The listing builds one solid part. Answer for the finished solid, in the listing's coordinates (mm). Round coordinates to 2 decimals unless told otherwise and drop trailing zeros. Order: outer loops, then holes, each group sorted by start corner. A loop starts at its lowest first (then second) coordinate and runs counter-clockwise, first axis right, second up. Notation, with made-up numbers: (32.25, -14) -> (75.25, -14) arc R20 ccw to (75.25, 19) -> close; hole circle Ø7 at (-9, 10.25). An arc over 180 degrees is marked (long way). Answer in a Markdown table with one row per item. Add a question column.
Autodesk Inventor part; units mm, degrees
ref_plane "YZ Plane" through (0, 0, 0) normal (1, 0, 0) x (0, 1, 0)
ref_plane "XZ Plane" through (0, 0, 0) normal (0, 1, 0) x (-1, 0, 0)
ref_plane "XY Plane" through (0, 0, 0) normal (0, 0, 1) x (1, 0, 0)
sketch "Sketch1" plane through (0, 0, 0) normal (0, 0, 1) x (1, 0, 0)
  line L0 (93.85, -64.2699) -> (-93.85, -64.2699)
  line L1 (-93.85, -64.2699) -> (-93.85, 55.2301)
  line L2 (-93.85, 55.2301) -> (93.85, 55.2301)
  line L3 (93.85, 55.2301) -> (93.85, -64.2699)
  line L4 (93.85, -64.2699) -> (-93.85, 55.2301) construction
  line L5 (-93.85, -64.2699) -> (93.85, 55.2301) construction
  point P0 (0, 0)
  point P1 (0, -4.5199)
  dimension "d0" = 187.7
  dimension "d1" = 119.5
extrude "Extrusion1" add sketch "Sketch1" along normal mid plane 2.5
hole "Hole2" at (-88.85, -59.3199, 1.25) direction (0, 0, -1) diameter 4 end through all countersink diameter 7 countersink angle 90
hole "Hole3" at (0, -59.2699, 1.25) direction (0, 0, -1) diameter 4 end through all countersink diameter 7 countersink angle 90
hole "Hole4" at (88.9, -59.2699, 1.25) direction (0, 0, -1) diameter 4 end through all countersink diameter 7 countersink angle 90
hole "Hole5" at (-88.9, 50.2301, 1.25) direction (0, 0, -1) diameter 4 end through all countersink diameter 7 countersink angle 90
hole "Hole6" at (0, 50.2301, 1.25) direction (0, 0, -1) diameter 4 end through all countersink diameter 7 countersink angle 90
hole "Hole7" at (88.9, 50.2301, 1.25) direction (0, 0, -1) diameter 4 end through all countersink diameter 7 countersink angle 90
hole "Hole8" at (76.35, -38.2699, 1.25) direction (0, 0, -1) diameter 4 end through all
hole "Hole9" at (76.35, 30.7301, 1.25) direction (0, 0, -1) diameter 4 end through all
hole "Hole10" at (-75.65, -38.2699, 1.25) direction (0, 0, -1) diameter 4 end through all
hole "Hole11" at (-75.65, 30.7301, 1.25) direction (0, 0, -1) diameter 4 end through all
sketch "Sketch5" plane through (0, 0, 1.25) normal (0, 0, 1) x (1, 0, 0)
  circle A0 centre (76.35, -38.2699) radius 2
  line L0 (93.85, -64.2699) -> (93.85, 55.2301)
  line L1 (-0.65, -21.7699) -> (85.35, -21.7699)
  line L2 (85.35, -21.7699) -> (85.35, -32.7699)
  line L3 (85.35, -32.7699) -> (-0.65, -32.7699)
  line L4 (-0.65, -32.7699) -> (-0.65, -21.7699)
  point P0 (0, 0)
  dimension "d120" = 8.5
  dimension "d121" = 5.5
  dimension "d122" = 11
  dimension "d123" = 86
extrude "Cut1" cut sketch "Sketch5" along normal through all both and the other way through all contours L1 L2 L3 L4
pattern_linear "Rectangular Pattern1" count 2 spacing 45.5 along (0, 1, 0) of "Cut1"
sketch "Sketch6" plane through (0, 0, 1.25) normal (0, 0, 1) x (1, 0, 0)
  line L0 (85.35, 23.7301) -> (85.35, 12.7301)
  line L1 (85.35, 12.7301) -> (-0.65, 12.7301)
  line L2 (5.85, 43.4801) -> (78.85, 43.4801)
  line L3 (78.85, 43.4801) -> (78.85, 33.2301)
  line L4 (78.85, 33.2301) -> (5.85, 33.2301)
  line L5 (5.85, 33.2301) -> (5.85, 43.4801)
  line L6 (-0.65, 23.7301) -> (-0.65, 12.7301)
  line L7 (-0.65, 12.7301) -> (85.35, 12.7301)
  line L8 (85.35, 12.7301) -> (85.35, 23.7301)
  line L9 (85.35, 23.7301) -> (-0.65, 23.7301)
  line L10 (-0.65, -21.7699) -> (-0.65, -32.7699)
  line L11 (-0.65, -32.7699) -> (85.35, -32.7699)
  line L12 (85.35, -32.7699) -> (85.35, -21.7699)
  line L13 (85.35, -21.7699) -> (-0.65, -21.7699)
  circle A0 centre (-75.65, 30.7301) radius 2
  circle A1 centre (-75.65, -38.2699) radius 2
  circle A2 centre (76.35, 30.7301) radius 2
  circle A3 centre (76.35, -38.2699) radius 2
  line L14 (-93.85, -64.2699) -> (-93.85, 55.2301)
  line L15 (-93.85, 55.2301) -> (93.85, 55.2301)
  line L16 (93.85, 55.2301) -> (93.85, -64.2699)
  line L17 (93.85, -64.2699) -> (-93.85, -64.2699)
  circle A4 centre (-88.85, -59.3199) radius 3.5
  circle A5 centre (0, -59.2699) radius 3.5
  circle A6 centre (88.9, -59.2699) radius 3.5
  circle A7 centre (-88.9, 50.2301) radius 3.5
  circle A8 centre (0, 50.2301) radius 3.5
  circle A9 centre (88.9, 50.2301) radius 3.5
  point P0 (0, 0)
  dimension "d129" = 6.5
  dimension "d130" = 20.5
  dimension "d131" = 73
  dimension "d132" = 10.25
extrude "Cut2" cut sketch "Sketch6" against normal through all contours L2 L3 L4 L5
hole "Hole12" at (5.85, 43.4801, 1.25) direction (0, 0, -1) diameter 3 end through all
hole "Hole13" at (78.85, 43.4801, 1.25) direction (0, 0, -1) diameter 3 end through all
hole "Hole14" at (5.85, 33.2301, 1.25) direction (0, 0, -1) diameter 3 end through all
hole "Hole16" at (78.85, 33.2301, 1.25) direction (0, 0, -1) diameter 3 end through all
hole "Hole17" at (-0.65, 23.7301, 1.25) direction (0, 0, -1) diameter 3 end through all
hole "Hole18" at (-0.65, 12.7301, 1.25) direction (0, 0, -1) diameter 3 end through all
hole "Hole19" at (85.35, 12.7301, 1.25) direction (0, 0, -1) diameter 3 end through all
hole "Hole20" at (85.35, 23.7301, 1.25) direction (0, 0, -1) diameter 3 end through all
hole "Hole21" at (-0.65, -21.7699, 1.25) direction (0, 0, -1) diameter 3 end through all
hole "Hole22" at (-0.65, -32.7699, 1.25) direction (0, 0, -1) diameter 3 end through all
hole "Hole23" at (85.35, -21.7699, 1.25) direction (0, 0, -1) diameter 3 end through all
hole "Hole24" at (85.35, -32.7699, 1.25) direction (0, 0, -1) diameter 3 end through all
equation "\"d124\" = Thickness"
equation "\"d133\" = Thickness"
equation "\"d142\" = Thickness"
equation "\"d151\" = Thickness"
equation "\"d160\" = Thickness"
equation "\"d178\" = Thickness"
equation "\"d187\" = Thickness"
equation "\"d196\" = Thickness"
equation "\"d205\" = Thickness"
equation "\"d214\" = Thickness"
equation "\"d223\" = Thickness"
equation "\"d232\" = Thickness"
equation "\"d241\" = Thickness"
equation "\"d250\" = Thickness"
equation "\"BendRadius\" = Thickness"
equation "\"BendReliefWidth\" = Thickness"
equation "\"BendReliefDepth\" = 0.5 * Thickness"
equation "\"CornerReliefSize\" = 4 * Thickness"
equation "\"MinimumRemnant\" = 2 * Thickness"
equation "\"TransitionRadius\" = BendRadius"
equation "\"JacobiRadiusSize\" = Thickness"
equation "\"GapSize\" = Thickness"
properties part number "Driver4BusV11Top"
1. The mould has two halves that part along Y. Classify faces 1 (the flat face through (-1, -4, 1.25)), 2 (the cylindrical face through (78.124, 29.807, -0.018)): released by +Y, released by -Y, zero draft, split by the parting line, or undercut.
2. The part is cut by section B-B (y = 18). Give the vertices of the cut face in (x, z), then the cut area to 3 significant figures.
3. The part is cut by section C-C (x = -75.65). Give the vertices of the cut face in (y, z), then the cut area to 3 significant figures.
4. Each of these flat-tipped pins is pushed along its axis until it touches: pin 1 (3.5 mm diameter, centred on x = -88.85, y = -59.32, fed in from -Z); pin 2 (4 mm diameter, centred on x = -0.65, y = -32.77, fed in from +Z); pin 3 (4.5 mm diameter, centred on x = 0, y = 50.23, fed in from +Z). Where does it stop, or does it pass through?
5. Straight lines are drawn through the part: line 1 along Y through (x, z) = (65.5, 1.1); line 2 along Y through (x, z) = (-75.65, -0.3); line 3 along Y through (x, z) = (0, -1). For each, find the intervals that lie inside material, in ascending order.
6. The part is cut by section D-D (x = 88.9). Give the vertices of the cut face in (y, z).
7. The part is cut by section A-A (x = 45). Give the vertices of the cut face in (y, z).
Report:
| question | item | result |
|---|---|---|
| 1 | face 1 | zero draft |
| 1 | face 2 | undercut |
| 2 | outline | (-93.85, -1.25) -> (-0.65, -1.25) -> (-0.65, 1.25) -> (-93.85, 1.25) -> close; (85.35, -1.25) -> (93.85, -1.25) -> (93.85, 1.25) -> (85.35, 1.25) -> close |
| 2 | area | 254 mm^2 |
| 3 | outline | (-64.27, -1.25) -> (-40.27, -1.25) -> (-40.27, 1.25) -> (-64.27, 1.25) -> close; (-36.27, -1.25) -> (28.73, -1.25) -> (28.73, 1.25) -> (-36.27, 1.25) -> close; (32.73, -1.25) -> (55.23, -1.25) -> (55.23, 1.25) -> (32.73, 1.25) -> close |
| 3 | area | 279 mm^2 |
| 4 | pin 1 | passes through |
| 4 | pin 2 | stops at z = 1.25 |
| 4 | pin 3 | stops at z = 0 |
| 5 | line 1 | y = -64.27 to -32.77, -21.77 to 12.73, 23.73 to 33.23, 43.48 to 55.23 |
| 5 | line 2 | y = -64.27 to -40.27, -36.27 to 28.73, 32.73 to 55.23 |
| 5 | line 3 | y = -64.27 to -61.27, -57.27 to -34.12, -20.42 to 11.38, 25.08 to 48.23, 52.23 to 55.23 |
| 6 | outline | (-64.27, -1.25) -> (-61.27, -1.25) -> (-61.27, -0.25) -> (-62.77, 1.25) -> (-64.27, 1.25) -> close; (-57.27, -1.25) -> (48.23, -1.25) -> (48.23, -0.25) -> (46.73, 1.25) -> (-55.77, 1.25) -> (-57.27, -0.25) -> close; (52.23, -1.25) -> (55.23, -1.25) -> (55.23, 1.25) -> (53.73, 1.25) -> (52.23, -0.25) -> close |
| 7 | outline | (-64.27, -1.25) -> (-32.77, -1.25) -> (-32.77, 1.25) -> (-64.27, 1.25) -> close; (-21.77, -1.25) -> (12.73, -1.25) -> (12.73, 1.25) -> (-21.77, 1.25) -> close; (23.73, -1.25) -> (33.23, -1.25) -> (33.23, 1.25) -> (23.73, 1.25) -> close; (43.48, -1.25) -> (55.23, -1.25) -> (55.23, 1.25) -> (43.48, 1.25) -> close |
